Build history of the part. All positions in model axes, mm. Coordinates: 2 decimals unless noted, no trailing zeros. Order: outer loops, then holes, each group sorted by start corner. A loop starts at its lowest first (then second) coordinate and runs counter-clockwise, first axis right, second up. Notation, with made-up numbers: (49.5, 4.5) - (96.5, 4.5) arc R22 ccw to (96.5, 21.5) - close; hole circle Ø11 at (0.5, -4.75). An arc over 180 degrees is marked (long way). Return JSON: item names as keys, results as strings.
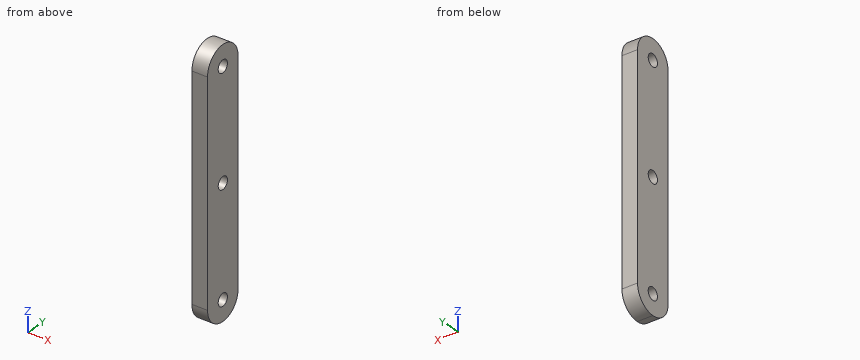
from build123d import *

# Parameters (mm, degrees)
SKETCH1_R                   = 16.66875
BOSS_EXTRUDE1_DEPTH         = 12.7
F_3_8_CLEARANCE_HOLE1_D     = 10.0838
F_3_8_CLEARANCE_HOLE1_DEPTH = 12.7
F_3_8_CLEARANCE_HOLE1_TIP   = 3.029479155


with BuildPart() as part:
    # Sketch1 → Boss-Extrude1 (new body)
    with BuildSketch(Plane(origin=(0, 0, 0), x_dir=(0, 0, -1), z_dir=(1, 0, 0))):
        with Locations((-88.9, 0)):
            Circle(SKETCH1_R)
        with BuildLine():
            Line((88.9, 16.66875), (-88.9, 16.66875))
            ThreePointArc((-88.9, 16.66875), (-77.113413841, 11.786586159), (-72.23125, 0))
            ThreePointArc((-72.23125, 0), (-77.113413841, -11.786586159), (-88.9, -16.66875))
            Line((-88.9, -16.66875), (88.9, -16.66875))
            ThreePointArc((88.9, -16.66875), (72.23125, 0), (88.9, 16.66875))
        make_face()
        with BuildLine():
            ThreePointArc((105.56875, 0), (100.686586159, 11.786586159), (88.9, 16.66875))
            Line((88.9, 16.66875), (88.9, -16.66875))
            ThreePointArc((88.9, -16.66875), (100.686586159, -11.786586159), (105.56875, 0))
        make_face()
        with BuildLine():
            Line((88.9, -16.66875), (88.9, 16.66875))
            ThreePointArc((88.9, 16.66875), (72.23125, 0), (88.9, -16.66875))
        make_face()
    extrude(amount=BOSS_EXTRUDE1_DEPTH)

    # 3/8 Clearance Hole1
    with Locations(Plane(origin=(12.7, 0, 0), x_dir=(0, 0, -1), z_dir=(1, 0, 0))):
        with Locations((0, 0), (88.9, 0), (-88.9, 0)):
            Hole(F_3_8_CLEARANCE_HOLE1_D / 2, depth=F_3_8_CLEARANCE_HOLE1_DEPTH)
            with Locations((0, 0, -(F_3_8_CLEARANCE_HOLE1_DEPTH + F_3_8_CLEARANCE_HOLE1_TIP / 2))):  # 118° drill point
                Cone(0, F_3_8_CLEARANCE_HOLE1_D / 2, F_3_8_CLEARANCE_HOLE1_TIP, mode=Mode.SUBTRACT)


solid = part.part
1. Drop a flat-ended pin along its axis: pin 1 (1.5 mm diameter, centred on x = 7, y = -4, fed in from -Z). Give the stop position or say it passes through.
Check values:
{"pin 1": "z = -105.25"}
2. Cut at A-A on z = 0. Give the cut face in (x, y), plus the area to 3 significant figures.
Check values:
{"outline": "(0, -16.67) - (12.7, -16.67) - (12.7, -5.04) - (0, -5.04) - close; (0, 5.04) - (12.7, 5.04) - (12.7, 16.67) - (0, 16.67) - close", "area": "295 mm²"}
3. Cut at D-D on y = -12.5. Give the cut face in (x, z).
Check values:
{"outline": "(0, -99.93) - (12.7, -99.93) - (12.7, 99.93) - (0, 99.93) - close"}
4. Cut at B-B on x = 6.5. Give the cut face in (y, z), plus the area to 3 significant figures.
Check values:
{"outline": "(-16.67, -88.9) arc R16.67 ccw to (16.67, -88.9) - (16.67, 88.9) arc R16.67 ccw to (-16.67, 88.9) - close; hole circle Ø10.08 at (0, -88.9); hole circle Ø10.08 at (0, 0); hole circle Ø10.08 at (0, 88.9)", "area": "6,560 mm²"}
5. Probe L1, parallel to Y at x = 4.25, z = -88.9; L2, parallel to Z at x = 6.75, y = -3.5; L3, parallel to Z at x = 4, y = -2. List the from-to ranges inside material, lowest first.
Check values:
{"L1": "-16.67 to -5.04, 5.04 to 16.67", "L2": "-105.2 to -92.53, -85.27 to -3.63, 3.63 to 85.27, 92.53 to 105.2", "L3": "-105.45 to -93.53, -84.27 to -4.63, 4.63 to 84.27, 93.53 to 105.45"}
6. Cut at C-C on y = 3. Give the cut face in (x, z), plus the area to 3 significant figures.
Check values:
{"outline": "(0, -105.3) - (12.7, -105.3) - (12.7, -92.95) - (0, -92.95) - close; (0, -84.85) - (12.7, -84.85) - (12.7, -4.05) - (0, -4.05) - close; (0, 4.05) - (12.7, 4.05) - (12.7, 84.85) - (0, 84.85) - close; (0, 92.95) - (12.7, 92.95) - (12.7, 105.3) - (0, 105.3) - close", "area": "2,370 mm²"}
